Study the drawing (mm; zero at the part's minimum x, y, z) and answer. A direction names the side the tool comes from. Give positions to 0.01 mm unless a question says otherwise; leave off trailing zeros. Write each loop counter-clockwise with the first axis right and the second up, starting at its lowest first coordinate (ties: lowest second). Pieces come first, ordered by that corner, then holes. Notation, with made-up numbers: M 31,64 L 75,64 A12 cw 75,68 Z; hole C 52,6.5 d2. An arc over 180 degrees is marked long. Use a Markdown table: item, result. Add a question column.
Item 1: Given P1, Ø4, axis at x = 6.5, y = 4.5, coming from the -Z side, flat-ended and moving along its own axis, determine where the tip first touches the part or whether it passes through.
Item 2: A cutting plane is placed at A-A on y = 9.5. Determine the outline of the cut face in (x, z), then the cut area to 3 significant figures.
Item 3: A cutting plane is placed at D-D on z = 14.75. Determine the outline of the cut face in (x, y), then the cut area to 3 significant figures.
Item 4: The mould has two halves that part along X. Classify the marked faces 3, 4, 5 and 6: pulls with the +X half, pulls with the -X half, needs draft (parallel to the pull), parting line crosses it, or undercut.
Item 5: Consider probe 1 along Z at (x, y) = (2.5, 1.75); probe 2 along X at (y, z) = (1.25, 8); probe 3 along Y at (x, z) = (13.5, 13.7). Determine where each line is inside the solid, lowest interval first. Write a range as [from, to].
Item 6: For the marked faces 1 and 2, determine the directions among +Z, -Z, +X, -X, +Y, -Y from which every point of the face is accessible in a straight line to the end or side of a thin tool.
Item 7: A cutting plane is placed at C-C on x = 6.5. Determine the outline of the cut face in (y, z).
Item 8: A cutting plane is placed at B-B on y = 4.5. Determine the outline of the cut face in (x, z), then the cut area to 3 significant figures.
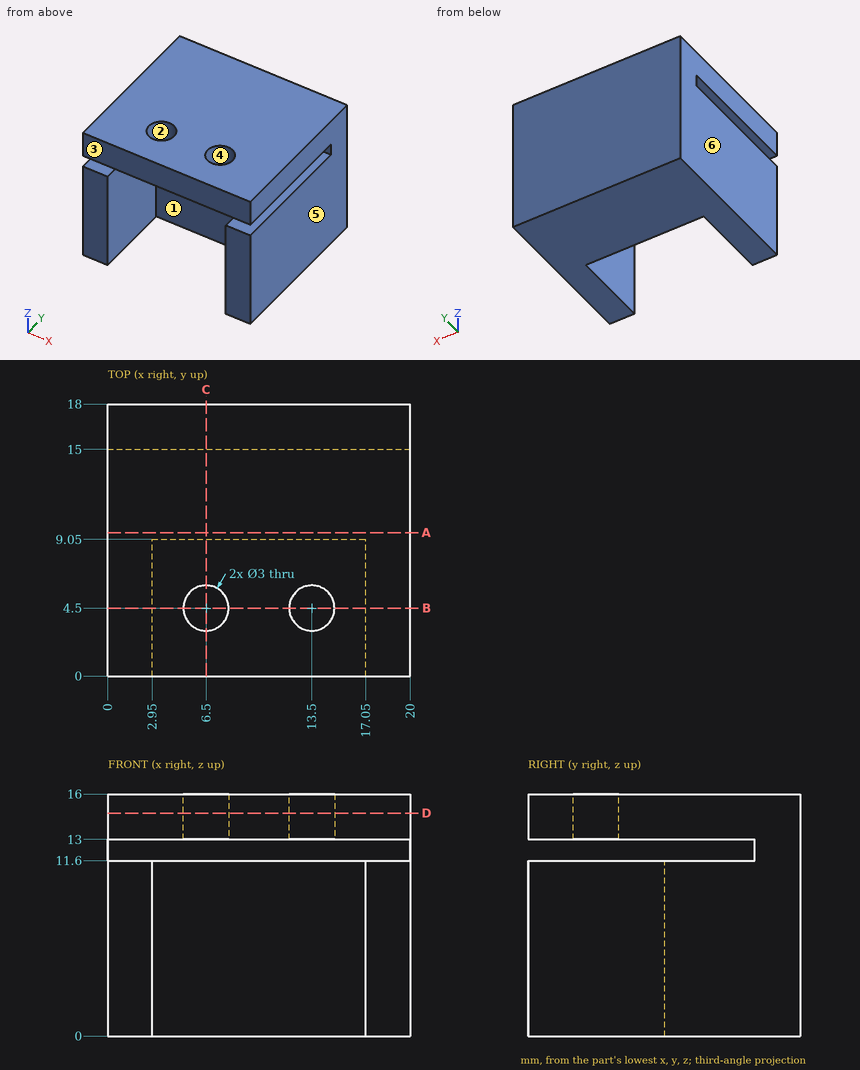
Filled in:
| question | item | result |
|---|---|---|
| 1 | P1 | z = 13 |
| 2 | outline | M 0,0 L 20,0 L 20,11.6 L 0,11.6 Z; M 0,13 L 20,13 L 20,16 L 0,16 Z |
| 2 | area | 292 mm² |
| 3 | outline | M 0,0 L 20,0 L 20,18 L 0,18 Z; hole C 6.5,4.5 d3; hole C 13.5,4.5 d3 |
| 3 | area | 346 mm² |
| 4 | face 3 | needs draft |
| 4 | face 4 | undercut |
| 4 | face 5 | pulls with the +X half |
| 4 | face 6 | pulls with the -X half |
| 5 | probe 1 | [0, 11.6], [13, 16] |
| 5 | probe 2 | [0, 2.95], [17.05, 20] |
| 5 | probe 3 | [0, 3], [6, 18] |
| 6 | face 1 | -Z, -Y |
| 6 | face 2 | +Z, -Z |
| 7 | outline | M 0,13 L 3,13 L 3,16 L 0,16 Z; M 6,13 L 15,13 L 15,11.6 L 9.05,11.6 L 9.05,0 L 18,0 L 18,16 L 6,16 Z |
| 8 | outline | M 0,0 L 2.95,0 L 2.95,11.6 L 0,11.6 Z; M 0,13 L 5,13 L 5,16 L 0,16 Z; M 8,13 L 12,13 L 12,16 L 8,16 Z; M 15,13 L 20,13 L 20,16 L 15,16 Z; M 17.05,0 L 20,0 L 20,11.6 L 17.05,11.6 Z |
| 8 | area | 110 mm² |
